Geometry: final body of the model. Coordinates: model frame, mm. Coordinates: 2 decimals unless noted, no trailing zeros. Write each loop counter-clockwise with the first axis right and the second up, starting at its lowest first coordinate (ties: lowest second). Pieces come first, ordered by that corner, then holes. Notation, with made-up numbers: (-21, 61.25) - (29, 61.25) arc R13 cw to (29, 81.25) - close; hole circle Ø8 at (-24, 86.5). An arc over 180 degrees is marked (long way). Put each result on its own line as item: value.
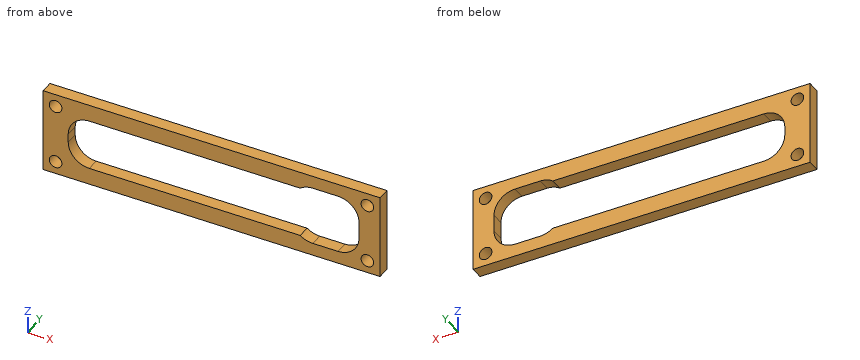
```python
from build123d import *

# Parameters (mm, degrees)
SKETCH1_W           = 80.213910902
SKETCH1_H           = 20
SKETCH1_R           = 1.5
SKETCH1_W_2         = 68.213910902
SKETCH1_H_2         = 12
BOSS_EXTRUDE1_DEPTH = 3
CUT_EXTRUDE1_DEPTH  = 83.724068458
FILLET1_R           = 5


with BuildPart() as part:
    # Sketch1 → Boss-Extrude1 (new body)
    with BuildSketch(Plane(origin=(0, 0, 0), x_dir=(1, 0, 0), z_dir=(0, 1, 0))):
        with Locations((40.106955451, 10)):
            Rectangle(SKETCH1_W, SKETCH1_H)
        with Locations(Location((3, 17, 0), (0, 0, 270))):
            Circle(SKETCH1_R, mode=Mode.SUBTRACT)
        with Locations(Location((3, 3, 0), (0, 0, 90))):
            Circle(SKETCH1_R, mode=Mode.SUBTRACT)
        with Locations(Location((77.213910902, 3, 0), (0, 0, 270))):
            Circle(SKETCH1_R, mode=Mode.SUBTRACT)
        with Locations(Location((77.213910902, 17, 0), (0, 0, 90))):
            Circle(SKETCH1_R, mode=Mode.SUBTRACT)
        with Locations((40.106955451, 10)):
            Rectangle(SKETCH1_W_2, SKETCH1_H_2, mode=Mode.SUBTRACT)
    extrude(amount=BOSS_EXTRUDE1_DEPTH)

    # Sketch2 → Cut-Extrude1 (cut, through all)
    with BuildSketch(Plane(origin=(0, 3, 0), x_dir=(1, 0, 0), z_dir=(0, 1, 0))):
        Polygon((61.213910902, 17), (61.213910902, 16), (74.213910902, 16), (74.213910902, 4), (61.213910902, 4), (61.213910902, 3), (75.213910902, 3), (75.213910902, 17), align=None)
    extrude(amount=-CUT_EXTRUDE1_DEPTH, mode=Mode.SUBTRACT)

    # Fillet1
    # the kernel refuses this fillet: 5 mm, written as the material it adds along each edge
    with BuildSketch(Plane(origin=(75.213910902, 3, -17), x_dir=(0, 0, 1), z_dir=(0, -1, 0)), Plane(origin=(75.213910902, 3, -3), x_dir=(-1, 0, 0), z_dir=(0, -1, 0)), Plane(origin=(6, 0, -16), x_dir=(0, 0, 1), z_dir=(0, 1, 0))) as fillet1_piece_1:
        with BuildLine():
            CenterArc((FILLET1_R, FILLET1_R), FILLET1_R, 180, 90)
            Line((0, FILLET1_R), (-FILLET1_R * 0.02, FILLET1_R))
            Line((-FILLET1_R * 0.02, FILLET1_R), (-FILLET1_R * 0.02, -FILLET1_R * 0.02))
            Line((-FILLET1_R * 0.02, -FILLET1_R * 0.02), (FILLET1_R, -FILLET1_R * 0.02))
            Line((FILLET1_R, -FILLET1_R * 0.02), (FILLET1_R, 0))
        make_face()
    extrude(amount=3)
    with BuildSketch(Plane(origin=(61.213910902, 3, -17), x_dir=(1, 0, 0), z_dir=(0, -1, 0))) as fillet1_piece_2:
        with BuildLine():
            CenterArc((3, 5), FILLET1_R, 233.130102354, 36.869897646)
            Line((0, 1), (-0.06, 0.92))
            ThreePointArc((-0.06, 0.92), (-0.1, 0.5), (-0.1, 0))
            Line((-0.1, 0), (0, -0.1))
            Line((0, -0.1), (3, -0.1))
            Line((3, -0.1), (3, 0))
        make_face()
    extrude(amount=3)
    with BuildSketch(Plane(origin=(61.213910902, 3, -3), x_dir=(0, 0, -1), z_dir=(0, -1, 0))) as fillet1_piece_3:
        with BuildLine():
            CenterArc((5, 3), FILLET1_R, 180, 36.869897646)
            Line((0, 3), (-0.1, 3))
            Line((-0.1, 3), (-0.1, 0))
            Line((-0.1, 0), (0, -0.1))
            ThreePointArc((0, -0.1), (0.5, -0.1), (0.92, -0.06))
            Line((0.92, -0.06), (1, 0))
        make_face()
    extrude(amount=3)
    with BuildSketch(Plane(origin=(6, 0, -4), x_dir=(0, 0, -1), z_dir=(0, 1, 0))) as fillet1_piece_4:
        with BuildLine():
            CenterArc((FILLET1_R, -FILLET1_R), FILLET1_R, 90, 90)
            Line((0, -FILLET1_R), (-FILLET1_R * 0.02, -FILLET1_R))
            Line((-FILLET1_R * 0.02, -FILLET1_R), (-FILLET1_R * 0.02, FILLET1_R * 0.02))
            Line((-FILLET1_R * 0.02, FILLET1_R * 0.02), (FILLET1_R, FILLET1_R * 0.02))
            Line((FILLET1_R, FILLET1_R * 0.02), (FILLET1_R, 0))
        make_face()
    extrude(amount=3)


solid = part.part
```
1. Pin query (flat end, axial travel): pin 1 Ø2.5 at (x, z) = (77.21, -17) entering from -Y. Return the tip coordinate at first contact, or that it passes through.
Answer below:
pin 1: passes through
2. Section query D-D (y = 1). Return loops of the section in (x, z).
Answer below:
outline: (0, -20) - (80.21, -20) - (80.21, 0) - (0, 0) - close; hole circle Ø3 at (3, -17); hole circle Ø3 at (3, -3); hole (6, -11) arc R5 ccw to (11, -16) - (61.21, -16) arc R5 ccw to (64.21, -17) - (70.21, -17) arc R5 ccw to (75.21, -12) - (75.21, -8) arc R5 ccw to (70.21, -3) - (64.21, -3) arc R5 ccw to (61.21, -4) - (11, -4) arc R5 ccw to (6, -9) - close; hole circle Ø3 at (77.21, -17); hole circle Ø3 at (77.21, -3)
3. Ray query, probe 1 along Z at (x, y) = (21.5, 2.45); probe 2 along Z at (x, y) = (68, 1.8); probe 3 along X at (y, z) = (2, -5.25). Return the intervals inside material, ascending. Write a range as from..to.
Answer below:
probe 1: z = -20..-16, -4..0
probe 2: z = -20..-17, -3..0
probe 3: x = 0..7.69, 74.39..80.21
4. Section query A-A (x = 3). Return loops of the section in (y, z).
Answer below:
outline: (0, -20) - (3, -20) - (3, -18.5) - (0, -18.5) - close; (0, -15.5) - (3, -15.5) - (3, -4.5) - (0, -4.5) - close; (0, -1.5) - (3, -1.5) - (3, 0) - (0, 0) - close
5. Section query B-B (x = 23). Return loops of the section in (y, z), then the cut area to 3 significant figures.
Answer below:
outline: (0, -20) - (3, -20) - (3, -16) - (0, -16) - close; (0, -4) - (3, -4) - (3, 0) - (0, 0) - close
area: 24.0 mm²
6. Section query C-C (z = -13.25). Return loops of the section in (x, y), then the cut area to 3 significant figures.
Answer below:
outline: (0, 0) - (6.53, 0) - (6.53, 3) - (0, 3) - close; (75.06, 0) - (80.21, 0) - (80.21, 3) - (75.06, 3) - close
area: 35.1 mm²
